Job drawing, mm, ordinate dimensions from the low corner. One solid piece. A direction names the side the tool comes from. Coordinates: 2 decimals unless noted, no trailing zeros. Order: outer loops, then holes, each group sorted by start corner. A loop starts at its lowest first (then second) coordinate and runs counter-clockwise, first axis right, second up. Notation, with made-up numbers: (88.5, 56.25) - (119.5, 56.25) arc R17 ccw to (119.5, 63.25) - close; hole circle Ø6 at (-14.5, 67.25). An arc over 180 degrees is marked (long way). Return JSON: item names as keys, results as strings.
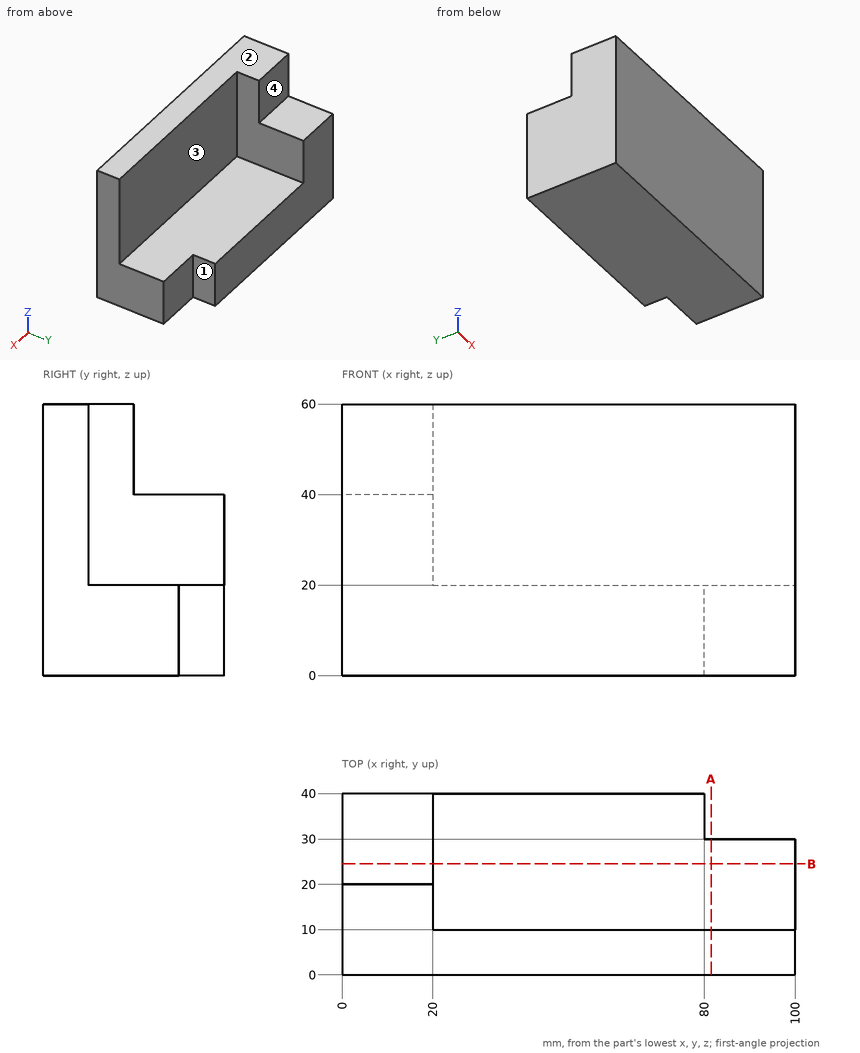
1. Probe L1, parallel to Y at x = 67, z = 34.5; L2, parallel to Z at x = 58, y = 23. List the from-to ranges inside material, lowest first.
Check values:
{"L1": "0 to 10", "L2": "0 to 20"}
2. Drop flat-ended pins along their axis: pin 1 (6 mm diameter, centred on x = 94.5, z = 10.5, fed in from +Y); pin 2 (9 mm diameter, centred on x = 52.5, y = 27, fed in from +Z); pin 3 (9 mm diameter, centred on y = 25, z = 49, fed in from +X); pin 4 (10 mm diameter, centred on x = 7.5, z = 47.5, fed in from +Y). Give the stop position or say it passes through.
Check values:
{"pin 1": "y = 30", "pin 2": "z = 20", "pin 3": "through", "pin 4": "y = 20"}
3. Cut at A-A on x = 81.5. Give the cut face in (y, z).
Check values:
{"outline": "(0, 0) - (30, 0) - (30, 20) - (10, 20) - (10, 60) - (0, 60) - close"}
4. Cut at B-B on y = 24.5. Give the cut face in (x, z).
Check values:
{"outline": "(0, 0) - (100, 0) - (100, 20) - (20, 20) - (20, 40) - (0, 40) - close"}
5. Tool access for the marked faces 1, 2, 3 and 4: list every direction of +Z, -Z, +X, -X, +Y, -Y with a clear straight run to the whole face (end or side of a thin tool).
Check values:
{"face 1": "+Z, -Z, +X, +Y", "face 2": "+Z, +X, -X, +Y, -Y", "face 3": "+Z, +X, +Y", "face 4": "+Z, +X, -X, +Y"}
